from build123d import *

# Parameters (mm, degrees)
SKETCH2_W           = 101.6
SKETCH2_H           = 101.6
BOSS_EXTRUDE1_DEPTH = 8.255
SKETCH3_W           = 97.536
SKETCH3_H           = 97.536
CUT_EXTRUDE1_DEPTH  = 6.223
SKETCH4_R           = 3.311109117
CUT_EXTRUDE2_DEPTH  = 2.032
SKETCH8_W           = 2.54
SKETCH8_H           = 0.762
CUT_EXTRUDE3_DEPTH  = 114.891812809


with BuildPart() as part:
    # Sketch2 → Boss-Extrude1 (new body)
    with BuildSketch(Plane.XY):
        Rectangle(SKETCH2_W, SKETCH2_H)
    extrude(amount=BOSS_EXTRUDE1_DEPTH)

    # Sketch3 → Cut-Extrude1 (cut)
    with BuildSketch(Plane(origin=(0, 0, 0), x_dir=(-1, 0, 0), z_dir=(0, 0, -1))):
        Rectangle(SKETCH3_W, SKETCH3_H)
    extrude(amount=-CUT_EXTRUDE1_DEPTH, mode=Mode.SUBTRACT)

    # Sketch4 → Cut-Extrude2 (cut)
    with BuildSketch(Plane.XY.offset(8.255)):
        with Locations((-37.456490902, 0)):
            Circle(SKETCH4_R)
    extrude(amount=-CUT_EXTRUDE2_DEPTH, mode=Mode.SUBTRACT)

    # Sketch8 → Cut-Extrude3 (cut, through all)
    with BuildSketch(Plane(origin=(50.8, 0, 0), x_dir=(0, 0, -1), z_dir=(1, 0, 0))):
        with Locations((-1.27, 50.419)):
            Rectangle(SKETCH8_W, SKETCH8_H)
    extrude(amount=-CUT_EXTRUDE3_DEPTH, mode=Mode.SUBTRACT)


solid = part.part
The listing builds one solid part. Answer for the finished solid, in the listing's coordinates (mm). A direction names the side the tool comes from. Round coordinates to 2 decimals unless told otherwise and drop trailing zeros. Write each loop counter-clockwise with the first axis right and the second up, starting at its lowest first coordinate (ties: lowest second). Pieces come first, ordered by that corner, then holes. Notation, with made-up numbers: M -22,12 L 26,12 A18 cw 26,38 Z; hole C -38.75,-15 d5. An arc over 180 degrees is marked long. Write each question's results on one line, items separated by ' | '. Start each with the question number.
Item 1: Flat-ended cylindrical pins translate along their axes: pin 1 Ø2 at (x, y) = (-16, -1.5) entering from -Z; pin 2 Ø2 at (x, z) = (21, 1.5) entering from +Y; pin 3 Ø7.5 at (x, y) = (-37.46, 0) entering from +Z (3 decimals). Find the tip coordinate at first contact, or state that the pin passes through.
Item 2: For a pull along Y with two mould halves and no side action, classify faces 4 (the face through (-1, -50.8, 4)), 5 (the face through (-1, 50.8, 5)), 6 (the face through (-48.768, -1, 3)) as pulls with the +Y half, pulls with the -Y half, needs draft (parallel to the pull), parting line crosses it, or undercut.
Item 3: A cutting plane is placed at B-B on z = 4.5. Write down the section's boundary in (x, y).
Item 4: A cutting plane is placed at D-D on y = -11.5. Write down the section's boundary in (x, z) (3 decimals).
Item 5: For faces 1 (the face through (-40.764, 0.146, 7.253)), 2 (the face through (1, 50.038, 1)), 3 (the face through (1, 48.768, 3)), determine the directions among +Z, -Z, +X, -X, +Y, -Y from which every point of the face is accessible in a straight line to the end or side of a thin tool.
Item 6: A cutting plane is placed at A-A on y = 0. Write down the section's boundary in (x, z) (3 decimals), and give its area (3 significant figures).
Item 7: Straight lines are drawn through the part: L1, parallel to Y at x = 31, z = 5.75; L2, parallel to Y at x = -34, z = 0.5. For each, find the intervals that lie inside material, in ascending order. Write a range as [from, to].
Item 8: A cutting plane is placed at C-C on x = 32. Write down the section's boundary in (y, z) (3 decimals).
Check sheet entries:
1) pin 1: z = 6.22 | pin 2: y = 50.04 | pin 3: z = 8.255
2) face 4: pulls with the -Y half | face 5: pulls with the +Y half | face 6: undercut
3) outline: M -50.8,-50.8 L 50.8,-50.8 L 50.8,50.8 L -50.8,50.8 Z; hole M -48.77,-48.77 L 48.77,-48.77 L 48.77,48.77 L -48.77,48.77 Z
4) outline: M -50.8,0 L -48.768,0 L -48.768,6.223 L 48.768,6.223 L 48.768,0 L 50.8,0 L 50.8,8.255 L -50.8,8.255 Z
5) face 1: +Z, -Z | face 2: -Z, +X, -X, +Y | face 3: -Z
6) outline: M -50.8,0 L -48.768,0 L -48.768,6.223 L -40.768,6.223 L -40.768,8.255 L -50.8,8.255 Z; M -34.145,6.223 L 48.768,6.223 L 48.768,0 L 50.8,0 L 50.8,8.255 L -34.145,8.255 Z | area: 218 mm²
7) L1: [-50.8, -48.77], [48.77, 50.8] | L2: [-50.8, -48.77], [48.77, 50.04]
8) outline: M -50.8,0 L -48.768,0 L -48.768,6.223 L 48.768,6.223 L 48.768,0 L 50.038,0 L 50.038,2.54 L 50.8,2.54 L 50.8,8.255 L -50.8,8.255 Z
